```python
from build123d import *

# Parameters (mm, degrees)
F1_DEPTH = 50
F3_DEPTH = 5
F6_DEPTH = 15


with BuildPart() as f1:
    # F0 (on Top) → F1 (new body, symmetric)
    with BuildSketch(Plane.XY):
        Polygon((0, -555), (0, 0), (-15, 0), (-15, -570), (-5, -570), (-5, -555), align=None)
    extrude(amount=F1_DEPTH, both=True)

    # F2 (on face) → F3 (cut)
    with BuildSketch(Plane.YZ):
        Polygon((-435.2, 34.8), (-435.2, -50), (-420, -50), (-420, 34.8), (0, 34.8), (0, 50), (-555, 50), (-555, 34.8), align=None)
    extrude(amount=-F3_DEPTH, mode=Mode.SUBTRACT)

    # F4: F1 across face


with BuildPart() as f1_1:
    add(f1.part)
    add(f1.part.mirror(Plane(origin=(-7.766854, 0, -2.262921), x_dir=(-1, 0, 0), z_dir=(0, 1, 0))))

    # F5 (on face) → F6 (cut, through all)
    with BuildSketch(Plane.YZ):
        with BuildLine():
            Line((-478.2, -20), (-478.2, -37))
            ThreePointArc((-478.2, -37), (-477.32132, -39.12132), (-475.2, -40))
            Line((-475.2, -40), (-458.2, -40))
            ThreePointArc((-458.2, -40), (-456.07868, -39.12132), (-455.2, -37))
            Line((-455.2, -37), (-455.2, -20))
            ThreePointArc((-455.2, -20), (-456.07868, -17.87868), (-458.2, -17))
            Line((-458.2, -17), (-475.2, -17))
            ThreePointArc((-475.2, -17), (-477.32132, -17.87868), (-478.2, -20))
        make_face()
    extrude(amount=-F6_DEPTH, mode=Mode.SUBTRACT)


solid = f1_1.part
```
Part model, mm, in its own coordinate system. Give positions to 0.01 mm unless a question says otherwise; leave off trailing zeros. Order: outer loops, then holes, each group sorted by start corner. A loop starts at its lowest first (then second) coordinate and runs counter-clockwise, first axis right, second up. Notation, with made-up numbers: M 10.25,-25 L 35.25,-25 A18 cw 35.25,3 Z; hole C -11,41 d9. An arc over 180 degrees is marked long. Use a Markdown table: item, result. Add a question column.
(1) Saw through at B-B, the plane y = 387. Give the cut face in (x, z).
(2) Saw through at A-A, the plane z = 0. Give the cut face in (x, y), and give its area (3 significant figures).
(3) Drop flat-ended pins along their axis: P1, Ø4, axis at x = -2.5, y = 471.5, coming from the +Z side; P2, Ø5.5, axis at x = -2, z = -23.5, coming from the +Y side; P3, Ø1, axis at x = -3, z = 38.5, coming from the -Y side; P4, Ø5.5, axis at x = -2, z = -17, coming from the -Y side. Give the stop position or say it passes through.
(4) Probe line 1 along Y through (x, z) = (-1.5, 0); line 2 along Y through (x, z) = (-11.25, -33); line 3 along Y through (x, z) = (-1, -26). List the from-to ranges inside material, lowest first. Write a range as [from, to].
Answer key:
| question | item | result |
|---|---|---|
| 1 | outline | M -15,-50 L 0,-50 L 0,34.8 L -5,34.8 L -5,50 L -15,50 Z |
| 2 | outline | M -15,-570 L -5,-570 L -5,-555 L 0,-555 L 0,-435.2 L -5,-435.2 L -5,-420 L 0,-420 L 0,420 L -5,420 L -5,435.2 L 0,435.2 L 0,555 L -5,555 L -5,570 L -15,570 Z |
| 2 | area | 16,800 mm^2 |
| 3 | P1 | z = 34.8 |
| 3 | P2 | y = 555 |
| 3 | P3 | through |
| 3 | P4 | y = -555 |
| 4 | line 1 | [-555, -435.2], [-420, 420], [435.2, 555] |
| 4 | line 2 | [-570, -478.2], [-455.2, 570] |
| 4 | line 3 | [-555, -478.2], [-455.2, -435.2], [-420, 420], [435.2, 555] |
